Check sheet for the modelled part. Datum: model origin and axes. Units: mm. A direction names the side the tool comes from. Give positions to 0.01 mm unless a question says otherwise; leave off trailing zeros. Write each loop counter-clockwise with the first axis right and the second up, starting at its lowest first coordinate (ties: lowest second). Pieces come first, ordered by that corner, then holes. Notation, with made-up numbers: (82, 78) -> (123, 78) arc R21 ccw to (123, 112) -> close; hole circle Ø11 at (39, -29). An arc over 180 degrees is marked (long way). Return JSON: item names as keys, results as strings.
from build123d import *

# Parameters (mm, degrees)
BOSS_EXTRUDE1_DEPTH  = 1.75
MOUNTING_HOLES_REACH = 199.898
SKETCH2_R            = 4.4
SKETCH2_R_2          = 1.55


with BuildPart() as part:
    # Sketch1 → Boss-Extrude1 (new body)
    with BuildSketch(Plane(origin=(0, 0, 0), x_dir=(1, 0, 0), z_dir=(0, 1, 0))):
        with BuildLine():
            Line((8.477821861, 23.002750629), (74.17169656, 128.134926657))
            ThreePointArc((74.17169656, 128.134926657), (75.398161995, 129.019168104), (76.893033195, 128.792319049))
            ThreePointArc((76.893033195, 128.792319049), (146.155509718, 33.742658152), (125.569837037, -82.050082429))
            ThreePointArc((125.569837037, -82.050082429), (124.325699782, -82.909281411), (122.835734015, -82.652177522))
            Line((122.835734015, -82.652177522), (17.703557987, -16.958302822))
            ThreePointArc((17.703557987, -16.958302822), (16.473932566, -16.661618944), (15.312221901, -17.162047094))
            ThreePointArc((15.312221901, -17.162047094), (-22.41051149, -5.17387425), (6.239187615, 22.137582025))
            ThreePointArc((6.239187615, 22.137582025), (7.502699505, 22.197060619), (8.477821861, 23.002750629))
        make_face()
        with BuildLine():
            Line((22.260126283, 10.270675628), (133.165216263, 35.875133138))
            ThreePointArc((133.165216263, 35.875133138), (134.43775302, 36.807406666), (134.638724504, 38.372045344))
            ThreePointArc((134.638724504, 38.372045344), (113.97617257, 81.2984138), (80.115562712, 114.810699028))
            ThreePointArc((80.115562712, 114.810699028), (78.570737863, 115.130073284), (77.274958481, 114.230384713))
            Line((77.274958481, 114.230384713), (16.958302822, 17.703557987))
            ThreePointArc((16.958302822, 17.703557987), (16.661618944, 16.473932566), (17.162047094, 15.312221901))
            ThreePointArc((17.162047094, 15.312221901), (18.724656922, 13.356167981), (20.06540624, 11.241862497))
            ThreePointArc((20.06540624, 11.241862497), (21.000901784, 10.390482389), (22.260126283, 10.270675628))
        make_face(mode=Mode.SUBTRACT)
        with BuildLine():
            Line((24.509636827, 0.52697498), (135.414726806, 26.131432491))
            ThreePointArc((135.414726806, 26.131432491), (136.967157083, 25.851353992), (137.833681508, 24.533166163))
            ThreePointArc((137.833681508, 24.533166163), (138.079984215, -23.10666482), (122.337088578, -68.070821636))
            ThreePointArc((122.337088578, -68.070821636), (121.08861366, -69.035079956), (119.529577356, -68.794477519))
            Line((119.529577356, -68.794477519), (23.002750629, -8.477821861))
            ThreePointArc((23.002750629, -8.477821861), (22.197060619, -7.502699505), (22.137582025, -6.239187615))
            ThreePointArc((22.137582025, -6.239187615), (22.684568835, -3.796094935), (22.96277582, -1.308023937))
            ThreePointArc((22.96277582, -1.308023937), (23.430373171, -0.132714311), (24.509636827, 0.52697498))
        make_face(mode=Mode.SUBTRACT)
    extrude(amount=BOSS_EXTRUDE1_DEPTH)

    # Sketch2 → Mounting_Holes (cut, up to next)
    with BuildSketch(Plane(origin=(0, 1.75, 0), x_dir=(1, 0, 0), z_dir=(0, 1, 0)), mode=Mode.PRIVATE) as mounting_holes_sk1:
        with Locations(Location((0, 0, 0), (0, 0, 270))):
            Circle(SKETCH2_R)
    mounting_holes_tool1 = extrude(mounting_holes_sk1.sketch, amount=-MOUNTING_HOLES_REACH, mode=Mode.PRIVATE) & part.part
    # Sketch2 → Mounting_Holes (cut, up to next)
    with BuildSketch(Plane(origin=(0, 1.75, 0), x_dir=(1, 0, 0), z_dir=(0, 1, 0)), mode=Mode.PRIVATE) as mounting_holes_sk2:
        with Locations(Location((8.064784864, 0, 0), (0, 0, 270))):
            Circle(SKETCH2_R_2)
    mounting_holes_tool2 = extrude(mounting_holes_sk2.sketch, amount=-MOUNTING_HOLES_REACH, mode=Mode.PRIVATE) & part.part
    # Sketch2 → Mounting_Holes (cut, up to next)
    with BuildSketch(Plane(origin=(0, 1.75, 0), x_dir=(1, 0, 0), z_dir=(0, 1, 0)), mode=Mode.PRIVATE) as mounting_holes_sk3:
        with Locations(Location((18.95, 0, 0), (0, 0, 270))):
            Circle(SKETCH2_R_2)
    mounting_holes_tool3 = extrude(mounting_holes_sk3.sketch, amount=-MOUNTING_HOLES_REACH, mode=Mode.PRIVATE) & part.part
    # Sketch2 → Mounting_Holes (cut, up to next)
    with BuildSketch(Plane(origin=(0, 1.75, 0), x_dir=(1, 0, 0), z_dir=(0, 1, 0)), mode=Mode.PRIVATE) as mounting_holes_sk4:
        with Locations(Location((-8.035215136, 0, 0), (0, 0, 270))):
            Circle(SKETCH2_R_2)
    mounting_holes_tool4 = extrude(mounting_holes_sk4.sketch, amount=-MOUNTING_HOLES_REACH, mode=Mode.PRIVATE) & part.part
    # Sketch2 → Mounting_Holes (cut, up to next)
    with BuildSketch(Plane(origin=(0, 1.75, 0), x_dir=(1, 0, 0), z_dir=(0, 1, 0)), mode=Mode.PRIVATE) as mounting_holes_sk5:
        with Locations(Location((0.014784864, 17.15, 0), (0, 0, 270))):
            Circle(SKETCH2_R_2)
    mounting_holes_tool5 = extrude(mounting_holes_sk5.sketch, amount=-MOUNTING_HOLES_REACH, mode=Mode.PRIVATE) & part.part
    # Sketch2 → Mounting_Holes (cut, up to next)
    with BuildSketch(Plane(origin=(0, 1.75, 0), x_dir=(1, 0, 0), z_dir=(0, 1, 0)), mode=Mode.PRIVATE) as mounting_holes_sk6:
        with Locations(Location((-0.014784864, -17.15, 0), (0, 0, 270))):
            Circle(SKETCH2_R_2)
    mounting_holes_tool6 = extrude(mounting_holes_sk6.sketch, amount=-MOUNTING_HOLES_REACH, mode=Mode.PRIVATE) & part.part
    # Sketch2 → Mounting_Holes (cut, up to next)
    with BuildSketch(Plane(origin=(0, 1.75, 0), x_dir=(1, 0, 0), z_dir=(0, 1, 0)), mode=Mode.PRIVATE) as mounting_holes_sk7:
        with Locations(Location((69.115919837, -43.188420035, 0), (0, 0, 270))):
            Circle(SKETCH2_R_2)
    mounting_holes_tool7 = extrude(mounting_holes_sk7.sketch, amount=-MOUNTING_HOLES_REACH, mode=Mode.PRIVATE) & part.part
    # Sketch2 → Mounting_Holes (cut, up to next)
    with BuildSketch(Plane(origin=(0, 1.75, 0), x_dir=(1, 0, 0), z_dir=(0, 1, 0)), mode=Mode.PRIVATE) as mounting_holes_sk8:
        with Locations(Location((122.966973943, -76.838293314, 0), (0, 0, 270))):
            Circle(SKETCH2_R_2)
    mounting_holes_tool8 = extrude(mounting_holes_sk8.sketch, amount=-MOUNTING_HOLES_REACH, mode=Mode.PRIVATE) & part.part
    # Sketch2 → Mounting_Holes (cut, up to next)
    with BuildSketch(Plane(origin=(0, 1.75, 0), x_dir=(1, 0, 0), z_dir=(0, 1, 0)), mode=Mode.PRIVATE) as mounting_holes_sk9:
        with Locations(Location((141.283659394, 32.61790288, 0), (0, 0, 270))):
            Circle(SKETCH2_R_2)
    mounting_holes_tool9 = extrude(mounting_holes_sk9.sketch, amount=-MOUNTING_HOLES_REACH, mode=Mode.PRIVATE) & part.part
    # Sketch2 → Mounting_Holes (cut, up to next)
    with BuildSketch(Plane(origin=(0, 1.75, 0), x_dir=(1, 0, 0), z_dir=(0, 1, 0)), mode=Mode.PRIVATE) as mounting_holes_sk10:
        with Locations(Location((79.41116028, 18.333510929, 0), (0, 0, 270))):
            Circle(SKETCH2_R_2)
    mounting_holes_tool10 = extrude(mounting_holes_sk10.sketch, amount=-MOUNTING_HOLES_REACH, mode=Mode.PRIVATE) & part.part
    # Sketch2 → Mounting_Holes (cut, up to next)
    with BuildSketch(Plane(origin=(0, 1.75, 0), x_dir=(1, 0, 0), z_dir=(0, 1, 0)), mode=Mode.PRIVATE) as mounting_holes_sk11:
        with Locations(Location((43.188420035, 69.115919837, 0), (0, 0, 270))):
            Circle(SKETCH2_R_2)
    mounting_holes_tool11 = extrude(mounting_holes_sk11.sketch, amount=-MOUNTING_HOLES_REACH, mode=Mode.PRIVATE) & part.part
    # Sketch2 → Mounting_Holes (cut, up to next)
    with BuildSketch(Plane(origin=(0, 1.75, 0), x_dir=(1, 0, 0), z_dir=(0, 1, 0)), mode=Mode.PRIVATE) as mounting_holes_sk12:
        with Locations(Location((76.838293314, 122.966973943, 0), (0, 0, 270))):
            Circle(SKETCH2_R_2)
    mounting_holes_tool12 = extrude(mounting_holes_sk12.sketch, amount=-MOUNTING_HOLES_REACH, mode=Mode.PRIVATE) & part.part
    add(mounting_holes_tool1.solids().sort_by_distance((0, 1.75, 0))[0], mode=Mode.SUBTRACT)
    add(mounting_holes_tool2.solids().sort_by_distance((8.064785, 1.75, 0))[0], mode=Mode.SUBTRACT)
    add(mounting_holes_tool3.solids().sort_by_distance((18.95, 1.75, 0))[0], mode=Mode.SUBTRACT)
    add(mounting_holes_tool4.solids().sort_by_distance((-8.035215, 1.75, 0))[0], mode=Mode.SUBTRACT)
    add(mounting_holes_tool5.solids().sort_by_distance((0.014785, 1.75, -17.15))[0], mode=Mode.SUBTRACT)
    add(mounting_holes_tool6.solids().sort_by_distance((-0.014785, 1.75, 17.15))[0], mode=Mode.SUBTRACT)
    add(mounting_holes_tool7.solids().sort_by_distance((69.11592, 1.75, 43.18842))[0], mode=Mode.SUBTRACT)
    add(mounting_holes_tool8.solids().sort_by_distance((122.966974, 1.75, 76.838293))[0], mode=Mode.SUBTRACT)
    add(mounting_holes_tool9.solids().sort_by_distance((141.283659, 1.75, -32.617903))[0], mode=Mode.SUBTRACT)
    add(mounting_holes_tool10.solids().sort_by_distance((79.41116, 1.75, -18.333511))[0], mode=Mode.SUBTRACT)
    add(mounting_holes_tool11.solids().sort_by_distance((43.18842, 1.75, -69.11592))[0], mode=Mode.SUBTRACT)
    add(mounting_holes_tool12.solids().sort_by_distance((76.838293, 1.75, -122.966974))[0], mode=Mode.SUBTRACT)


solid = part.part
(1) Cross-section at B-B on y = 0.65. State how many separate pieces and enclosed holes the cut face has, then the cut area to 3 significant figures.
Reply:
{"separate pieces": "1", "enclosed holes": "14", "area": "7,420 mm^2"}
(2) Depth check by flat-ended pin: pin 1 Ø1 at (x, y) = (47, 0.5) entering from +Z; pin 2 Ø3 at (x, z) = (-8.04, 0) entering from -Y. Enter the tip coordinate at first touch or a pass-through.
Reply:
{"pin 1": "z = 35.58", "pin 2": "through"}
(3) Thickness scan on L1, parallel to Z at x = 125, y = 1.05; L2, parallel to X at y = 0.55, z = 17.15; L3, parallel to Z at x = 53, y = 0.3. Record the ranges inside material, lowest first.
Reply:
{"L1": "-82.92 to -63.05, -33.99 to -23.73, 63.05 to 82.62", "L2": "-15.33 to -1.56, 1.54 to 15.33, 18.01 to 36.88, 138.95 to 149.02", "L3": "-94.25 to -75.38, -17.37 to -7.1, 27.22 to 39.01"}
(4) Release check for a two-part mould opening along X. For faces 1 (the flat face through (40.865, 0.863, -74.833)), 2 (the flat face through (77, 1.75, -16)), 3 (the flat face through (47.539, 0.863, -66.643)) record: pulls with the +X half, pulls with the -X half, needs draft (parallel to the pull), parting line crosses it, or undercut.
Reply:
{"face 1": "pulls with the -X half", "face 2": "needs draft", "face 3": "undercut"}
(5) Cross-section at A-A on z = 33.5. Enter the section's corners in (x, y), then the cut area to 3 significant figures.
Reply:
{"outline": "(44.18, 0) -> (63.05, 0) -> (63.05, 1.75) -> (44.18, 1.75) -> close; (135.93, 0) -> (146.21, 0) -> (146.21, 1.75) -> (135.93, 1.75) -> close", "area": "51.0 mm^2"}
(6) Cross-section at C-C on z = 11. Enter the section's corners in (x, y), then the cut area to 3 significant figures.
Reply:
{"outline": "(-20.2, 0) -> (27.04, 0) -> (27.04, 1.75) -> (-20.2, 1.75) -> close; (139.57, 0) -> (149.6, 0) -> (149.6, 1.75) -> (139.57, 1.75) -> close", "area": "100 mm^2"}
(7) Set-up check for faces 4 (the flat face through (71.942, 0.863, 39.058)), 5 (the flat face through (77, 0, -16)): record each of +Z, -Z, +X, -X, +Y, -Y from which the full face is reachable in a straight line by a thin tool's end or side.
Reply:
{"face 4": "+Y, -Y", "face 5": "+Z, -Z, +X, -X, -Y"}
